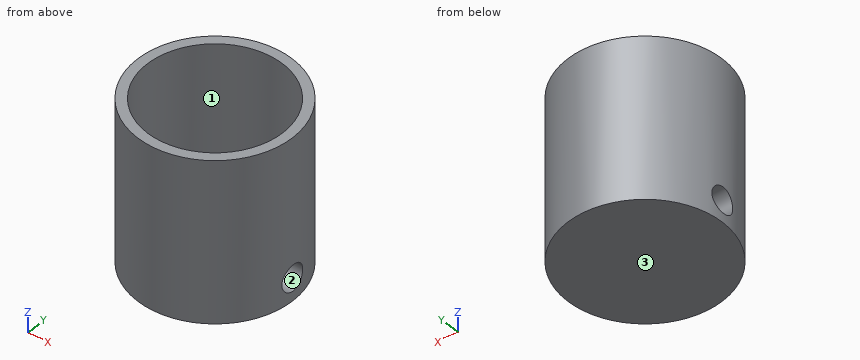
from build123d import *

# Parameters (mm, degrees)
F0_R     = 9.59
F0_R_2   = 8.39
F1_DEPTH = 15
F2_DEPTH = 1.2
F3_W     = 2
F3_H     = 6
F4_DEPTH = 5
F5_R     = 1.6
F6_DEPTH = 15.2727807522
F7_DEPTH = 5
F8_DEPTH = 5
F9_DEPTH = 39.7


with BuildPart() as f1:
    # F0 (on Top) → F1 (new body)
    with BuildSketch(Plane.XY):
        Circle(F0_R)
        Circle(F0_R_2, mode=Mode.SUBTRACT)
    extrude(amount=F1_DEPTH)

    # F0 (on Top) → F2 (join)
    with BuildSketch(Plane.XY):
        Circle(F0_R_2)
    extrude(amount=F2_DEPTH)

    # F3 (on face) → F4 (join)
    with BuildSketch(Plane.XY):
        with Locations((-4.6817807522, 0)):
            Rectangle(F3_W, F3_H)
        with Locations((4.6817807522, 0)):
            Rectangle(F3_W, F3_H)
    extrude(amount=-F4_DEPTH)

    # F5 (on face) → F6 (cut, through all)
    with BuildSketch(Plane.YZ.offset(5.6817807522)):
        with Locations((0, -2.223377116)):
            Circle(F5_R)
    extrude(amount=-F6_DEPTH, mode=Mode.SUBTRACT)

    # F0 (on Top) → F7 (join)
    with BuildSketch(Plane.XY):
        Circle(F0_R_2)
    extrude(amount=-F7_DEPTH)

    # F0 (on Top) → F8 (join)
    with BuildSketch(Plane.XY):
        Circle(F0_R)
        Circle(F0_R_2, mode=Mode.SUBTRACT)
    extrude(amount=-F8_DEPTH)

    # F5 (on face) → F9 (cut, symmetric)
    with BuildSketch(Plane.YZ.offset(5.6817807522)):
        with Locations((0, -2.223377116)):
            Circle(F5_R)
    extrude(amount=F9_DEPTH, both=True, mode=Mode.SUBTRACT)


solid = f1.part
Work out the finished part from the listing and answer in its coordinate system (mm). Face numbers are marked on the shaded views. Coordinates: 2 decimals unless noted, no trailing zeros. Loops run counter-clockwise (first coordinate to the right, second up) from the corner with the lowest first, then second, coordinate; pieces in that order, holes last. Notation, with made-up numbers: M 68.25,33.25 L 83.25,33.25 A25 cw 83.25,66.25 Z; hole C 44.25,55 d3. An arc over 180 degrees is marked long. Answer in a Markdown table with one row per item. Add a question column.
1. Find section C-C, the plane z = -3. Write down the section's boundary in (x, y), then the cut area to 3 significant figures.
2. Find section B-B, the plane x = -4. Write down the section's boundary in (y, z), then the cut area to 3 significant figures.
3. The mould has two halves that part along Z. Classify the marked faces 1, 2 and 3: pulls with the +Z half, pulls with the -Z half, needs draft (parallel to the pull), parting line crosses it, or undercut.
4. Find section D-D, the plane y = -7. Write down the section's boundary in (x, z) (3 decimals), then the cut area to 3 significant figures.
5. Find section A-A, the plane y = 0. Write down the section's boundary in (x, z), then the cut area to 3 significant figures.
6. Consider L1, parallel to Y at x = 0, z = 7.5; L2, parallel to Z at x = -1.5, y = -3; L3, parallel to Z at x = 3.5, y = 0. Determine where each line is inside the solid, lowest interval first.
7. Flat-ended cylindrical pins translate along their axes: P1, Ø3, axis at y = -3, z = 11, coming from the -X side; P2, Ø8.5, axis at x = -3, y = -0.5, coming from the +Z side; P3, Ø1, axis at x = 4, z = 6.5, coming from the +Y side. Find the tip coordinate at first contact, or state that the pin passes through.
Reported:
| question | item | result |
|---|---|---|
| 1 | outline | M -9.49,-1.4 A9.59 ccw 9.49,-1.4 Z; M -9.49,1.4 L 9.49,1.4 A9.59 ccw Z |
| 1 | area | 235 mm^2 |
| 2 | outline | M -8.72,-5 L 8.72,-5 L 8.72,15 L 7.38,15 L 7.38,1.2 L -7.38,1.2 L -7.38,15 L -8.72,15 Z; hole C 0,-2.22 d3.2 |
| 2 | area | 137 mm^2 |
| 3 | face 1 | needs draft |
| 3 | face 2 | undercut |
| 3 | face 3 | pulls with the -Z half |
| 4 | outline | M -6.555,-5 L 6.555,-5 L 6.555,15 L 4.625,15 L 4.625,1.2 L -4.625,1.2 L -4.625,15 L -6.555,15 Z |
| 4 | area | 135 mm^2 |
| 5 | outline | M -9.59,-5 L 9.59,-5 L 9.59,-3.82 L -9.59,-3.82 Z; M -9.59,-0.62 L 9.59,-0.62 L 9.59,15 L 8.39,15 L 8.39,1.2 L -8.39,1.2 L -8.39,15 L -9.59,15 Z |
| 5 | area | 90.7 mm^2 |
| 6 | L1 | y = -9.59 to -8.39, 8.39 to 9.59 |
| 6 | L2 | z = -5 to 1.2 |
| 6 | L3 | z = -5 to -3.82, -0.62 to 1.2 |
| 7 | P1 | stops at x = -9.47 |
| 7 | P2 | stops at z = 1.2 |
| 7 | P3 | stops at y = 8.93 |
